from build123d import *

# Parameters (mm, degrees)
SKETCH_1_R          = 1
EXTRUDE_1_DEPTH     = 2
CUT_EXTRUDE_START   = 1
SKETCH_1_8_R        = 1.75
SKETCH_1_8_R_2      = 1
CUT_EXTRUDE_2_DEPTH = 1


with BuildPart() as part:
    # 草图1 → 凸台-拉伸1 (new body)
    with BuildSketch(Plane.XY):
        Polygon((36.5, 0), (-6, 0), (-6, -19.5), (40.4, -19.5), (40.4, -10), (54.5, -10), (54.5, -1), (36.5, -1), align=None)
        with Locations((36.9, -13.5)):
            Circle(SKETCH_1_R, mode=Mode.SUBTRACT)
        with Locations((3, -2.5)):
            Circle(SKETCH_1_R, mode=Mode.SUBTRACT)
        with Locations((33.5, -2.5)):
            Circle(SKETCH_1_R, mode=Mode.SUBTRACT)
        with Locations((-3, -16.5)):
            Circle(SKETCH_1_R, mode=Mode.SUBTRACT)
        with Locations((15.4, -13.5)):
            Circle(SKETCH_1_R, mode=Mode.SUBTRACT)
        with Locations((52.2, -7.5)):
            Circle(SKETCH_1_R, mode=Mode.SUBTRACT)
    extrude(amount=EXTRUDE_1_DEPTH)

    # 草图1<8> → 切除-拉伸2 (cut)
    # profile 1 of 6: a face of its own
    with BuildSketch(Plane.XY.offset(CUT_EXTRUDE_START)):
        with Locations((52.2, -7.5)):
            Circle(SKETCH_1_8_R)
        with Locations((52.2, -7.5)):
            Circle(SKETCH_1_8_R_2, mode=Mode.SUBTRACT)
    # profile 2 of 6: a face of its own
    with BuildSketch(Plane.XY.offset(CUT_EXTRUDE_START)):
        with Locations((3, -2.5)):
            Circle(SKETCH_1_8_R)
    # profile 3 of 6: a face of its own
    with BuildSketch(Plane.XY.offset(CUT_EXTRUDE_START)):
        with Locations((33.5, -2.5)):
            Circle(SKETCH_1_8_R)
    # profile 4 of 6: a face of its own
    with BuildSketch(Plane.XY.offset(CUT_EXTRUDE_START)):
        with Locations((-3, -16.5)):
            Circle(SKETCH_1_8_R)
    # profile 5 of 6: a face of its own
    with BuildSketch(Plane.XY.offset(CUT_EXTRUDE_START)):
        with Locations((15.4, -13.5)):
            Circle(SKETCH_1_8_R)
    # profile 6 of 6: a face of its own
    with BuildSketch(Plane.XY.offset(CUT_EXTRUDE_START)):
        with Locations((36.9, -13.5)):
            Circle(SKETCH_1_8_R)
    extrude(amount=CUT_EXTRUDE_2_DEPTH, mode=Mode.SUBTRACT)


solid = part.part
Check sheet for the modelled part. Datum: model origin and axes. Units: mm. A direction names the side the tool comes from. Give positions to 0.01 mm unless a question says otherwise; leave off trailing zeros. Loops run counter-clockwise (first coordinate to the right, second up) from the corner with the lowest first, then second, coordinate; pieces in that order, holes last. Notation, with made-up numbers: M 4,36 L 36,36 A29 cw 36,72 Z; hole C 68,-25.5 d11. An arc over 180 degrees is marked long. Use a Markdown table: item, result. Add a question column.
Q1. Sectioned sample at D-D, the plane y = -13.5. Record the cut outline in (x, z), then the cut area to 3 significant figures.
Q2. Tool access check on faces 4 (the flat face through (46, -1, 1)), 5 (the flat face through (40.4, -15, 1)), 6 (the cylindrical face through (50.45, -7.42, 1.49)). Record the directions out of +Z, -Z, +X, -X, +Y, -Y that give a thin tool (end or side, any length) a straight path to the whole face; none if there is none.
Q3. Sectioned sample at C-C, the plane z = 0.4. Record the cut outline in (x, y).
Q4. Scan lines: line 1 along X through (y, z) = (-13.5, 0.6); line 2 along X through (y, z) = (-2.5, 0.7); line 3 along Y through (x, z) = (-3, 1.3). Record each from-to range of solid material in increasing order. Write a range as [from, to].
Q5. Go/stop test with flat-tipped pins: pin 1 (3 mm diameter, centred on x = -2.5, y = -16, fed in from +Z); pin 2 (1 mm diameter, centred on x = 44.5, z = 1, fed in from -Y); pin 3 (1.2 mm diameter, centred on x = 33.5, y = -2.5, fed in from +Z); pin 4 (1 mm diameter, centred on y = -13.5, z = 1, fed in from +X). Record where each tip stops, or that it passes through.
Q6. Sectioned sample at B-B, the plane x = 52.2. Record the cut outline in (y, z).
Q7. Sectioned sample at A-A, the plane y = -16.5. Record the cut outline in (x, z).
Q8. Mould release check, pull along Y, two halves, no side actions. Record for faces 1 (the cylindrical face through (51.463, -6.824, 0.493)), 2 (the flat face through (16, 0, 1)), 3 (the flat face through (54.5, -6, 1)): pulls with the +Y half, pulls with the -Y half, needs draft (parallel to the pull), parting line crosses it, or undercut.
Verdict:
| question | item | result |
|---|---|---|
| 1 | outline | M -6,0 L 14.4,0 L 14.4,1 L 13.65,1 L 13.65,2 L -6,2 Z; M 16.4,0 L 35.9,0 L 35.9,1 L 35.15,1 L 35.15,2 L 17.15,2 L 17.15,1 L 16.4,1 Z; M 37.9,0 L 40.4,0 L 40.4,2 L 38.65,2 L 38.65,1 L 37.9,1 Z |
| 1 | area | 81.8 mm^2 |
| 2 | face 4 | +Z, -Z, +X, +Y |
| 2 | face 5 | +Z, -Z, +X, -Y |
| 2 | face 6 | +Z |
| 3 | outline | M -6,-19.5 L 40.4,-19.5 L 40.4,-10 L 54.5,-10 L 54.5,-1 L 36.5,-1 L 36.5,0 L -6,0 Z; hole C -3,-16.5 d2; hole C 3,-2.5 d2; hole C 15.4,-13.5 d2; hole C 33.5,-2.5 d2; hole C 36.9,-13.5 d2; hole C 52.2,-7.5 d2 |
| 4 | line 1 | [-6, 14.4], [16.4, 35.9], [37.9, 40.4] |
| 4 | line 2 | [-6, 2], [4, 32.5], [34.5, 54.5] |
| 4 | line 3 | [-19.5, -18.25], [-14.75, 0] |
| 5 | pin 1 | z = 2 |
| 5 | pin 2 | y = -10 |
| 5 | pin 3 | through |
| 5 | pin 4 | x = 40.4 |
| 6 | outline | M -10,0 L -8.5,0 L -8.5,1 L -9.25,1 L -9.25,2 L -10,2 Z; M -6.5,0 L -1,0 L -1,2 L -5.75,2 L -5.75,1 L -6.5,1 Z |
| 7 | outline | M -6,0 L -4,0 L -4,1 L -4.75,1 L -4.75,2 L -6,2 Z; M -2,0 L 40.4,0 L 40.4,2 L -1.25,2 L -1.25,1 L -2,1 Z |
| 8 | face 1 | undercut |
| 8 | face 2 | pulls with the +Y half |
| 8 | face 3 | needs draft |
